from build123d import *

# Parameters (mm, degrees)
BOSS_EXTRUDE1_DEPTH = 2
CUT_EXTRUDE2_DEPTH  = 122.638809596
BOSS_EXTRUDE2_DEPTH = 1.2
CHAMFER1_SIZE       = 1.2
SKETCH2_R           = 1.65
CUT_EXTRUDE3_DEPTH  = 122.638809596
FILLET1_R           = 3


with BuildPart() as part:
    # Sketch1 → Boss-Extrude1 (new body)
    with BuildSketch(Plane.XY):
        with BuildLine():
            Line((-86, -7.75), (-86, -27.75))
            Line((-86, -27.75), (-80.567396197, -27.75))
            ThreePointArc((-80.567396197, -27.75), (-80.317201092, -27.765711107), (-80.07093683, -27.81259759))
            Line((-80.07093683, -27.81259759), (-41.814217278, -37.615881976))
            ThreePointArc((-41.814217278, -37.615881976), (-41.320172025, -37.815786012), (-40.896463083, -38.139070823))
            Line((-40.896463083, -38.139070823), (-38.139070823, -40.896463083))
            ThreePointArc((-38.139070823, -40.896463083), (-37.815786012, -41.320172025), (-37.615881976, -41.814217278))
            Line((-37.615881976, -41.814217278), (-27.81259759, -80.07093683))
            ThreePointArc((-27.81259759, -80.07093683), (-27.765711107, -80.317201092), (-27.75, -80.567396197))
            Line((-27.75, -80.567396197), (-27.75, -86))
            Line((-27.75, -86), (-7.75, -86))
            Line((-7.75, -86), (-7.75, -80.567396197))
            ThreePointArc((-7.75, -80.567396197), (-7.734288893, -80.317201092), (-7.68740241, -80.07093683))
            Line((-7.68740241, -80.07093683), (-4.385282287, -67.184614401))
            ThreePointArc((-4.385282287, -67.184614401), (-3.674069354, -66.101054981), (-2.447879878, -65.681073768))
            Line((-2.447879878, -65.681073768), (-1, -65.681073768))
            ThreePointArc((-1, -65.681073768), (0.414213562, -65.09528733), (1, -63.681073768))
            Line((1, -63.681073768), (1, -1))
            ThreePointArc((1, -1), (0.414213562, 0.414213562), (-1, 1))
            Line((-1, 1), (-63.681073768, 1))
            ThreePointArc((-63.681073768, 1), (-65.09528733, 0.414213562), (-65.681073768, -1))
            Line((-65.681073768, -1), (-65.681073768, -2.447879878))
            ThreePointArc((-65.681073768, -2.447879878), (-66.101054981, -3.674069354), (-67.184614401, -4.385282287))
            Line((-67.184614401, -4.385282287), (-80.07093683, -7.68740241))
            ThreePointArc((-80.07093683, -7.68740241), (-80.317201092, -7.734288893), (-80.567396197, -7.75))
            Line((-80.567396197, -7.75), (-86, -7.75))
        make_face()
    extrude(amount=BOSS_EXTRUDE1_DEPTH)

    # Sketch4 → Cut-Extrude2 (cut, through all)
    with BuildSketch(Plane.XY):
        with BuildLine():
            Line((-24.968684618, -12.968684618), (-24.968684618, -20.140257493))
            ThreePointArc((-24.968684618, -20.140257493), (-24.816443683, -20.905624358), (-24.38289818, -21.554471055))
            Line((-24.38289818, -21.554471055), (-21.554471055, -24.38289818))
            ThreePointArc((-21.554471055, -24.38289818), (-20.905624358, -24.816443683), (-20.140257493, -24.968684618))
            Line((-20.140257493, -24.968684618), (-12.968684618, -24.968684618))
            ThreePointArc((-12.968684618, -24.968684618), (-11.554471055, -24.38289818), (-10.968684618, -22.968684618))
            Line((-10.968684618, -22.968684618), (-10.968684618, -12.968684618))
            ThreePointArc((-10.968684618, -12.968684618), (-11.554471055, -11.554471055), (-12.968684618, -10.968684618))
            Line((-12.968684618, -10.968684618), (-22.968684618, -10.968684618))
            ThreePointArc((-22.968684618, -10.968684618), (-24.38289818, -11.554471055), (-24.968684618, -12.968684618))
        make_face()
    extrude(amount=CUT_EXTRUDE2_DEPTH, mode=Mode.SUBTRACT)

    # Sketch5 → Boss-Extrude2 (add)
    with BuildSketch(Plane.XY):
        with BuildLine():
            Line((-78.471636399, -9.961587833), (-46.073118848, -1.659467711))
            ThreePointArc((-46.073118848, -1.659467711), (-45.839167799, -1.614925552), (-45.601482449, -1.6))
            Line((-45.601482449, -1.6), (-3.5, -1.6))
            ThreePointArc((-3.5, -1.6), (-2.156497116, -2.156497116), (-1.6, -3.5))
            Line((-1.6, -3.5), (-1.6, -45.601482449))
            ThreePointArc((-1.6, -45.601482449), (-1.614925552, -45.839167799), (-1.659467711, -46.073118848))
            Line((-1.659467711, -46.073118848), (-9.961587833, -78.471636399))
            ThreePointArc((-9.961587833, -78.471636399), (-10.63724012, -79.501017848), (-11.802120122, -79.9))
            Line((-11.802120122, -79.9), (-23.697879878, -79.9))
            ThreePointArc((-23.697879878, -79.9), (-24.86275988, -79.501017848), (-25.538412167, -78.471636399))
            Line((-25.538412167, -78.471636399), (-35.267187197, -40.505685062))
            ThreePointArc((-35.267187197, -40.505685062), (-35.477086435, -39.986937546), (-35.816535486, -39.542043158))
            Line((-35.816535486, -39.542043158), (-39.542043158, -35.816535486))
            ThreePointArc((-39.542043158, -35.816535486), (-39.986937546, -35.477086435), (-40.505685062, -35.267187197))
            Line((-40.505685062, -35.267187197), (-78.471636399, -25.538412167))
            ThreePointArc((-78.471636399, -25.538412167), (-79.501017848, -24.86275988), (-79.9, -23.697879877))
            Line((-79.9, -23.697879877), (-79.9, -11.802120122))
            ThreePointArc((-79.9, -11.802120122), (-79.501017848, -10.63724012), (-78.471636399, -9.961587833))
        make_face()
        with BuildLine():
            Line((-77.8, -11.957332135), (-77.8, -23.542667865))
            Line((-77.8, -23.542667865), (-39.984402726, -33.232914667))
            ThreePointArc((-39.984402726, -33.232914667), (-38.946907695, -33.652713143), (-38.057118917, -34.331611246))
            Line((-38.057118917, -34.331611246), (-34.331611246, -38.057118917))
            ThreePointArc((-34.331611246, -38.057118917), (-33.652713143, -38.946907695), (-33.232914667, -39.984402726))
            Line((-33.232914667, -39.984402726), (-23.542667865, -77.8))
            Line((-23.542667865, -77.8), (-11.957332135, -77.8))
            Line((-11.957332135, -77.8), (-3.7, -45.57626484))
            Line((-3.7, -45.57626484), (-3.7, -3.7))
            Line((-3.7, -3.7), (-45.57626484, -3.7))
            Line((-45.57626484, -3.7), (-77.8, -11.957332135))
        make_face(mode=Mode.SUBTRACT)
    extrude(amount=-BOSS_EXTRUDE2_DEPTH)

    # Chamfer1
    chamfer1_edges = [part.edges().sort_by_distance(p)[0] for p in [
        (-28.387791266, -58.892201363, 0),
        (-33.652713143, -38.946907695, 0),
        (-36.194365081, -36.194365081, 0),
        (-38.946907695, -33.652713143, 0),
        (-17.75, -77.8, 0),
        (-7.828666067, -61.68813242, 0),
        (-3.7, -24.63813242, 0),
        (-24.63813242, -3.7, 0),
        (-61.68813242, -7.828666067, 0),
        (-77.8, -17.75, 0),
        (-58.892201363, -28.387791266, 0),
    ]]
    chamfer(chamfer1_edges, length=CHAMFER1_SIZE - 0.0001)  # a hair under: the kernel refuses the full size

    # Sketch2 → Cut-Extrude3 (cut, through all)
    with BuildSketch(Plane.XY):
        with Locations((-61.681073768, -2)):
            Circle(SKETCH2_R)
        with Locations((-2, -61.681073768)):
            Circle(SKETCH2_R)
    extrude(amount=CUT_EXTRUDE3_DEPTH, mode=Mode.SUBTRACT)

    # Fillet1
    fillet1_edges = [part.edges().sort_by_distance(p)[0] for p in [
        (-7.75, -86, 1),
        (-27.75, -86, 1),
        (-86, -27.75, 1),
        (-86, -7.75, 1),
    ]]
    fillet(fillet1_edges, radius=FILLET1_R)


solid = part.part
CAD build for the part. Positions are in the model's coordinates, mm. A direction names the side the tool comes from. Give positions to 0.01 mm unless a question says otherwise; leave off trailing zeros. Answer as CSV lines item,"result".
Q1. 3-axis set-ups, long thin cutter, end or side, ignore diameter. For faces 5 (the face through (-38.67, -33.13, -0.61)), 6 (the face through (-11.57, -24.4, 0.99)), 7 (the face through (-8.65, -85.14, 1.01)), 8 (the face through (-85.14, -26.85, 1.01)), 9 (the face through (-59.22, -30.47, -0.59)): which of +Z, -Z, +X, -X, +Y, -Y reach the whole face in a straight line?
Result set:
face 5,"-Z"
face 6,"+Z, -Z"
face 7,"+Z, -Z, +X, -Y"
face 8,"+Z, -Z, -X, -Y"
face 9,"-Z, -X, -Y"
Q2. Drill centre lines: line 1 (X direction, y = -14.5, z = 0.25); line 2 (X direction, y = -2, z = 1.3). Where is each one in solid material? Low to high. Write a range as from..to.
Result set:
line 1,"-86..-24.97, -10.97..1"
line 2,"-65.68..-63.33, -60.03..1"
Q3. Flat gauge pins, fed straight in: pin 1 Ø0.6 at (y, z) = (-82, 0.5) entering from -X; pin 2 Ø1.6 at (x, z) = (-81.5, 0.5) entering from +Y; pin 3 Ø1 at (x, z) = (-82, 0.5) entering from -Y. Where does each tip first touch, or does it go through?
Result set:
pin 1,"x = -27.75"
pin 2,"y = -7.75"
pin 3,"y = -27.75"
Q4. Band-saw the part on D-D (z = 1.35). State how many separate pieces and enclosed holes the cut face has, and give its area (3 significant figures).
Result set:
separate pieces,"1"
enclosed holes,"3"
area,"4,230 mm²"
Q5. Pull direction X, two halves, no side cores. Call faces 1 (the face through (-24.37, -11.54, 0.99)), 2 (the face through (-32.783, -60.675, 0.986)), 3 (the face through (-82, -7.75, 1)), 4 (the face through (-33.15, -38.64, -0.61)): released by +X, released by -X, zero draft, split by the parting line, or undercut.
Result set:
face 1,"undercut"
face 2,"released by -X"
face 3,"zero draft"
face 4,"undercut"
